Print and shaded views of the part. All mm, measured from the part's lowest x, y and z. Coordinates: 2 decimals unless noted, no trailing zeros. Loops run counter-clockwise (first coordinate to the right, second up) from the corner with the lowest first, then second, coordinate; pieces in that order, holes last. Notation, with made-up numbers: M 10,22 L 46,22 A15 cw 46,49 Z; hole C 12,17.5 d4. An arc over 180 degrees is marked long. Answer as CSV lines item,"result". Start each with the question number.
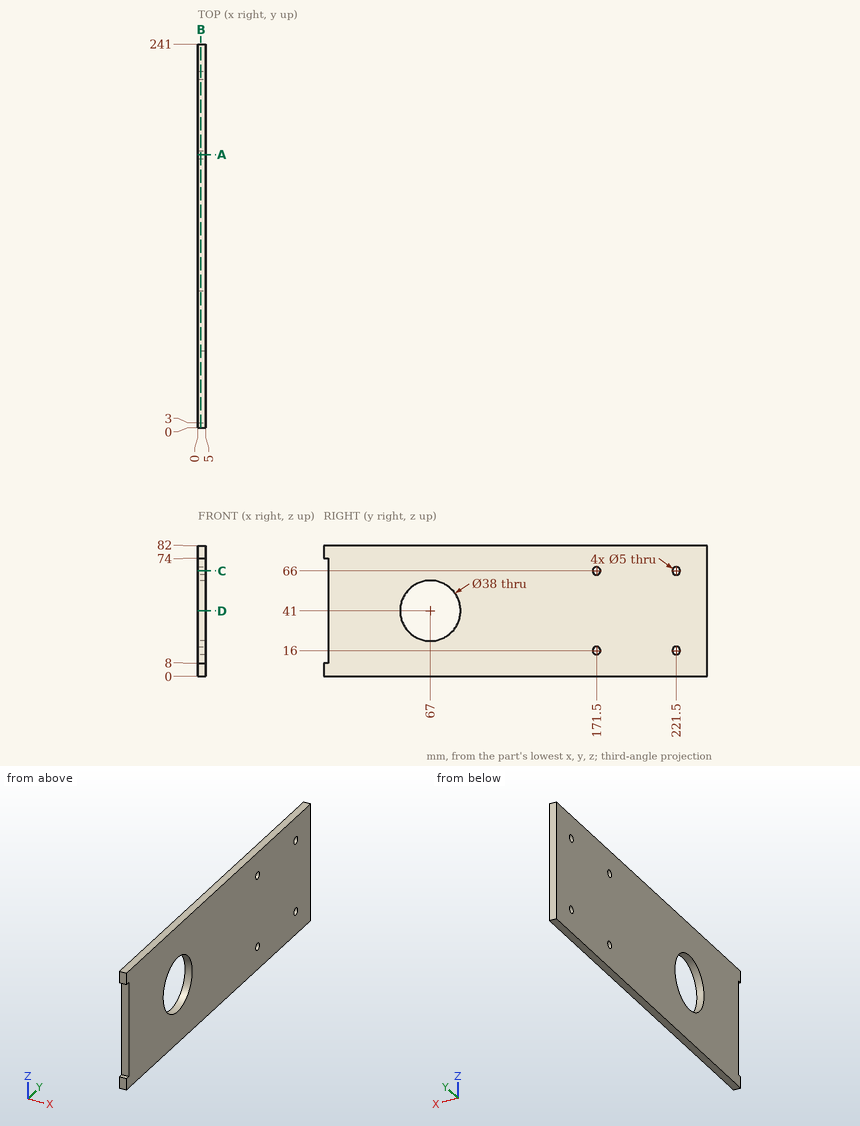
Q1. Slice it at B-B, the plane x = 1.9. Write the cut outline in (y, z), and give its area (3 significant figures).
Q2. Slice it at C-C, the plane z = 66. Write the cut outline in (x, y).
Q3. Slice it at D-D, the plane z = 41. Write the cut outline in (x, y), and give its area (3 significant figures).
Q4. Wall check: L1, parallel to Z at x = 4.7, y = 172; L2, parallel to Z at x = 1.35, y = 221.5; L3, parallel to Y at x = 0.85, z = 14.5. Give the ranges that are in metal, low to high.
Q5. Slice it at A-A, the plane y = 171.5. Write the cut outline in (x, z), and give its area (3 significant figures).
Solved:
1,outline,"M 0,0 L 241,0 L 241,82 L 0,82 L 0,74 L 3,74 L 3,8 L 0,8 Z; hole C 67,41 d38; hole C 171.5,16 d5; hole C 171.5,66 d5; hole C 221.5,16 d5; hole C 221.5,66 d5"
1,area,"18,400 mm2"
2,outline,"M 0,3 L 5,3 L 5,169 L 0,169 Z; M 0,174 L 5,174 L 5,219 L 0,219 Z; M 0,224 L 5,224 L 5,241 L 0,241 Z"
3,outline,"M 0,3 L 5,3 L 5,48 L 0,48 Z; M 0,86 L 5,86 L 5,241 L 0,241 Z"
3,area,"1,000 mm2"
4,L1,"z = 0 to 13.55, 18.45 to 63.55, 68.45 to 82"
4,L2,"z = 0 to 13.5, 18.5 to 63.5, 68.5 to 82"
4,L3,"y = 3 to 169.5, 173.5 to 219.5, 223.5 to 241"
5,outline,"M 0,0 L 5,0 L 5,13.5 L 0,13.5 Z; M 0,18.5 L 5,18.5 L 5,63.5 L 0,63.5 Z; M 0,68.5 L 5,68.5 L 5,82 L 0,82 Z"
5,area,"360 mm2"
